Build history of the part. All positions in model axes, mm. A direction names the side the tool comes from. Round coordinates to 2 decimals unless told otherwise and drop trailing zeros. Write each loop counter-clockwise with the first axis right and the second up, starting at its lowest first coordinate (ties: lowest second). Pieces come first, ordered by that corner, then holes.
1) Saw through at B-B (z = -18.5). Write the cut outline in (x, y), plus the area to 4 significant figures.
2) Which spindle directions (+Z, -Z, +X, -X, +Y, -Y) get a long thin tool onto all of the face, cutting with end or side? Do faces 4 (the flat face through (40, 15, -10)), 5 (the flat face through (25, 0, -15)), 6 (the flat face through (15, 35, -10)), 7 (the flat face through (50, 10, -11)), 8 (the flat face through (44, 20, -6)). Say none if no direction does.
3) Saw through at A-A (y = 34). Write the cut outline in (x, z).
4) Wall check: probe 1 along Y at (x, z) = (29.5, -14); probe 2 along Z at (x, y) = (14, 37); probe 3 along X at (y, z) = (11.5, -12.5). Give the ranges that are in metal, low to high.
5) Saw through at C-C (x = 38). Write the cut outline in (y, z).
6) Pull direction Z, two halves, no side cores. Call faces 1 (the flat face through (19, 15, 0)), 2 (the flat face through (16, 30, -15)), 3 (the flat face through (25, 40, -25)): +Z half, -Z half, draft (parallel to the pull), parting line (faces both ways), or undercut.
7) Saw through at D-D (z = -1.5). Write the cut outline in (x, y).
8) Flat gauge pins, fed straight in: pin 1 (2 mm diameter, centred on x = 24.5, z = -13, fed in from +Y); pin 2 (10 mm diameter, centred on x = 43.5, z = -10.5, fed in from +Y). Where does each tip first touch, or does it go through?
Autodesk Inventor part; units mm, degrees
ref_plane "YZ Plane" through (0, 0, 0) normal (1, 0, 0) x (0, 1, 0)
ref_plane "XZ Plane" through (0, 0, 0) normal (0, 1, 0) x (-1, 0, 0)
ref_plane "XY Plane" through (0, 0, 0) normal (0, 0, 1) x (1, 0, 0)
sketch "草圖1" plane through (0, 0, 0) normal (0, 1, 0) x (-1, 0, 0)
  line L0 (0, 0) -> (-50, 0)
  line L1 (-50, 0) -> (-50, -30)
  line L2 (-50, -30) -> (0, -30)
  line L3 (0, -30) -> (0, 0)
  dimension "d0" = 30
  dimension "d1" = 50
extrude "擠出1" add sketch "草圖1" along normal blind 40
sketch "草圖2" plane through (50, 0, 0) normal (1, 0, 0) x (0, 0, -1)
  line L0 (0, 40) -> (30, 40)
  line L1 (10, 40) -> (20, 40)
  line L2 (20, 40) -> (20, 30)
  line L3 (20, 30) -> (10, 30)
  line L4 (10, 30) -> (10, 40)
  point P0 (0, 0)
  dimension "d4" = 10
  dimension "d5" = 10
  dimension "d6" = 10
extrude "擠出2" cut sketch "草圖2" against normal through all
sketch "草圖3" plane through (0, 40, 0) normal (0, 1, 0) x (1, 0, 0)
  line L0 (50, 0) -> (50, 30)
  line L1 (50, 30) -> (20, 0)
  line L2 (0, 0) -> (50, 0)
  line L3 (50, 20) -> (30, 0)
  line L4 (20, 0) -> (30, 0)
  line L5 (50, 30) -> (50, 20)
  dimension "d9" = 10
  dimension "d10" = 135
extrude "擠出3" cut sketch "草圖3" against normal blind 30 contours L3 L2 L1 L0
sketch "草圖4" plane through (0, 40, 0) normal (0, 1, 0) x (1, 0, 0)
  line L0 (40, 10) -> (30, 0)
  line L1 (30, 0) -> (50, 0)
  line L2 (50, 0) -> (50, 10)
  line L3 (50, 10) -> (40, 10)
  line L4 (50, 20) -> (40, 10)
  line L5 (50, 10) -> (40, 10)
  line L6 (50, 20) -> (50, 10)
  point P0 (0, 0)
extrude "擠出4" cut sketch "草圖4" against normal blind 20
properties part number "17"
Evaluation:
1. outline: (0, 0) - (50, 0) - (50, 20) - (48.5, 20) - (48.5, 10) - (38.5, 10) - (38.5, 30) - (0, 30) - close
1. area: 1,285 mm2
2. face 4: +Y
2. face 5: +Z, -Z, +X, -X, -Y
2. face 6: +X, -X, +Y
2. face 7: +Z, -Z, +X, +Y, -Y
2. face 8: +Z, +X, +Y
3. outline: (0, -30) - (50, -30) - (40, -20) - (0, -20) - close; (0, -10) - (30, -10) - (20, 0) - (0, 0) - close
4. probe 1: y = 0 to 30
4. probe 2: z = -30 to -20, -10 to 0
4. probe 3: x = 0 to 32.5, 42.5 to 50
5. outline: (0, -30) - (40, -30) - (40, -20) - (30, -20) - (30, -18) - (10, -18) - (10, -8) - (20, -8) - (20, 0) - (0, 0) - close
6. face 1: +Z half
6. face 2: undercut
6. face 3: draft
7. outline: (0, 0) - (50, 0) - (50, 20) - (31.5, 20) - (31.5, 10) - (21.5, 10) - (21.5, 40) - (0, 40) - close
8. pin 1: stops at y = 30
8. pin 2: stops at y = 20
